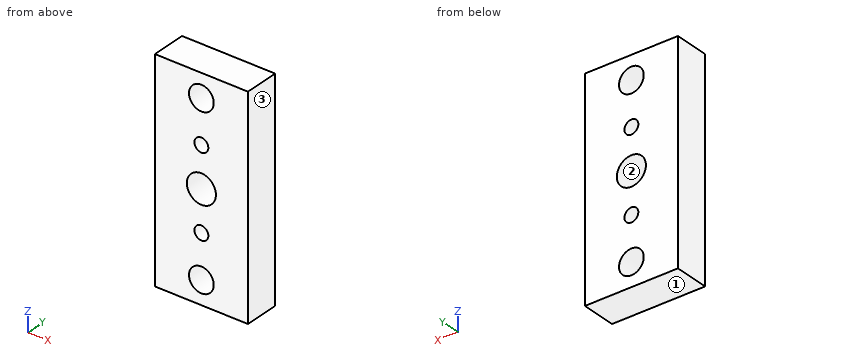
from build123d import *

# Parameters (mm, degrees)
SKETCH1_W                   = 25.4
SKETCH1_H                   = 9.525
EXTRUDE1_DEPTH              = 58.42
F_1_4_CLEARANCE_HOLE1_D     = 6.7564
F_1_4_CLEARANCE_HOLE1_DEPTH = 12.7
F_1_4_CLEARANCE_HOLE1_TIP   = 2.029827343
F_3_8_16_TAPPED_HOLE1_D     = 7.9375
F_10_24_TAPPED_HOLE1_D      = 3.7973
CIRPATTERN1_COUNT           = 2


with BuildPart() as part:
    # Sketch1 → Extrude1 (new body)
    with BuildSketch(Plane.XY):
        Rectangle(SKETCH1_W, SKETCH1_H)
    extrude(amount=EXTRUDE1_DEPTH)

    # 1/4 Clearance Hole1
    with Locations(Plane(origin=(0, 4.7625, 6.35), x_dir=(0, 0, 1), z_dir=(0, 1, 0))):
        with Locations((0, 0), (45.72, 0)):
            Hole(F_1_4_CLEARANCE_HOLE1_D / 2, depth=F_1_4_CLEARANCE_HOLE1_DEPTH)
            with Locations((0, 0, -(F_1_4_CLEARANCE_HOLE1_DEPTH + F_1_4_CLEARANCE_HOLE1_TIP / 2))):  # 118° drill point
                Cone(0, F_1_4_CLEARANCE_HOLE1_D / 2, F_1_4_CLEARANCE_HOLE1_TIP, mode=Mode.SUBTRACT)

    # 3/8-16 Tapped Hole1 (through all)
    with Locations(Plane(origin=(0, 4.7625, 29.21), x_dir=(0, 0, 1), z_dir=(0, 1, 0))):
        with Locations((0, 0)):
            Hole(F_3_8_16_TAPPED_HOLE1_D / 2)

    # #10-24 Tapped Hole1 (through all)
    with Locations(Plane(origin=(0, 4.7625, 40.259), x_dir=(0, 0, 1), z_dir=(0, 1, 0))):
        with Locations((0, 0)):
            f_10_24_tapped_hole1 = Hole(F_10_24_TAPPED_HOLE1_D / 2)

    # CirPattern1: #10-24 Tapped Hole1 ×2 about axis
    cirpattern1_axis = Axis((0, 0, 29.21), (0, 1, 0))
    for i in range(1, CIRPATTERN1_COUNT):
        add(f_10_24_tapped_hole1.rotate(cirpattern1_axis, i * 360 / CIRPATTERN1_COUNT), mode=Mode.SUBTRACT)


solid = part.part
For this review, take the finished solid that the model builds, in its own axes (mm). Face numbers are marked on the shaded views. Round coordinates to 2 decimals unless told otherwise and drop trailing zeros. Loops run counter-clockwise (first coordinate to the right, second up) from the corner with the lowest first, then second, coordinate; pieces in that order, holes last. Notation, with made-up numbers: (40, 44.25) - (72, 44.25) arc R8 cw to (72, 58.25) - close; hole circle Ø2 at (3.25, 75). An arc over 180 degrees is marked (long way). Use one line per item in the form item = value.
1) We need section A-A on z = 29.21. Write out the cut boundary in (x, y).
Solutions:
outline = (-12.7, -4.76) - (-3.97, -4.76) - (-3.97, 4.76) - (-12.7, 4.76) - close; (3.97, -4.76) - (12.7, -4.76) - (12.7, 4.76) - (3.97, 4.76) - close
2) Clearance check with a flat-ended pin moving along its axis: P1, Ø5, axis at x = 0, z = 18.161, coming from the +Y side. State where the tip first meets the part, or that it passes through.
Solutions:
P1 = 4.76
3) Wall thickness on probe 1 along X at (y, z) = (0.25, 6.35); probe 2 along Z at (x, y) = (3.5, 0); probe 3 along X at (y, z) = (-3, 4): over which ranges is each line inside the solid? List them lowest first.
Solutions:
probe_1 = -12.7 to -3.38, 3.38 to 12.7
probe_2 = 0 to 27.34, 31.08 to 58.42
probe_3 = -12.7 to -2.43, 2.43 to 12.7
4) We need section D-D on z = 6.35. Write out the cut boundary in (x, y).
Solutions:
outline = (-12.7, -4.76) - (-3.38, -4.76) - (-3.38, 4.76) - (-12.7, 4.76) - close; (3.38, -4.76) - (12.7, -4.76) - (12.7, 4.76) - (3.38, 4.76) - close
5) We need section C-C on y = -3. Write out the cut boundary in (x, z), then the cut area to 3 significant figures.
Solutions:
outline = (-12.7, 0) - (12.7, 0) - (12.7, 58.42) - (-12.7, 58.42) - close; hole circle Ø7.94 at (0, 29.21); hole circle Ø6.76 at (0, 6.35); hole circle Ø6.76 at (0, 52.07); hole circle Ø3.8 at (0, 18.16); hole circle Ø3.8 at (0, 40.26)
area = 1,340 mm2
6) Mouldability with a two-part tool opening along Z and no side actions: class the marked faces 1, 2 and 3 as pulls with the +Z half, pulls with the -Z half, needs draft (parallel to the pull), parting line crosses it, or undercut.
Solutions:
face_1 = pulls with the -Z half
face_2 = undercut
face_3 = needs draft
7) We need section B-B on x = 0. Write out the cut boundary in (y, z), then the cut area to 3 significant figures.
Solutions:
outline = (-4.76, 0) - (4.76, 0) - (4.76, 2.97) - (-4.76, 2.97) - close; (-4.76, 9.73) - (4.76, 9.73) - (4.76, 16.26) - (-4.76, 16.26) - close; (-4.76, 20.06) - (4.76, 20.06) - (4.76, 25.24) - (-4.76, 25.24) - close; (-4.76, 33.18) - (4.76, 33.18) - (4.76, 38.36) - (-4.76, 38.36) - close; (-4.76, 42.16) - (4.76, 42.16) - (4.76, 48.69) - (-4.76, 48.69) - close; (-4.76, 55.45) - (4.76, 55.45) - (4.76, 58.42) - (-4.76, 58.42) - close
area = 280 mm2
